Study the drawing (mm; zero at the part's minimum x, y, z) and answer. A direction names the side the tool comes from. Coordinates: 2 decimals unless noted, no trailing zeros. Order: outer loops, then holes, each group sorted by start corner. A loop starts at its lowest first (then second) coordinate and runs counter-clockwise, first axis right, second up.
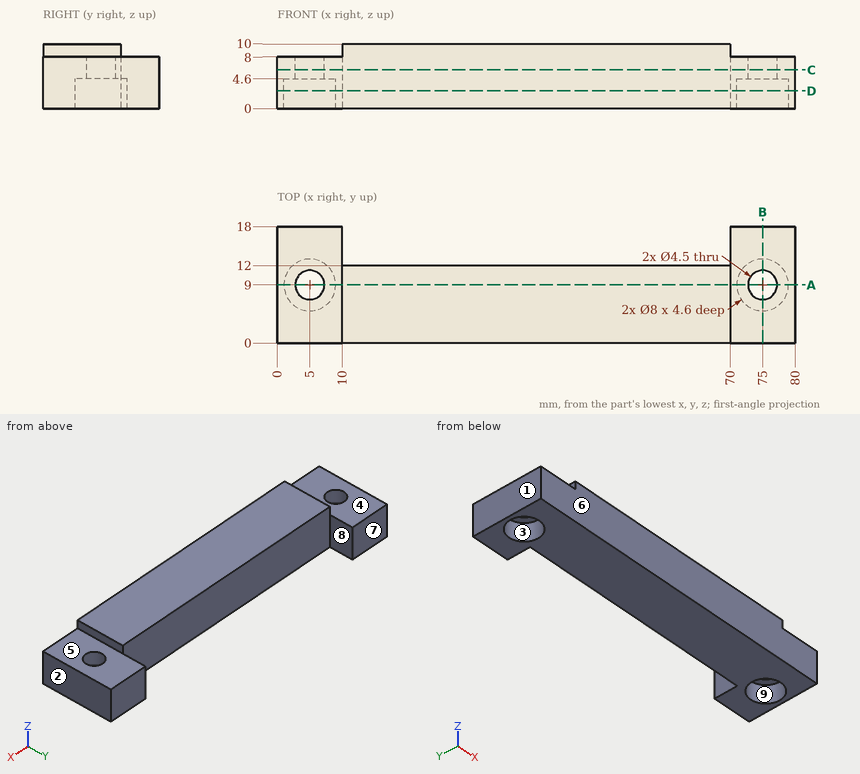
1) A cutting plane is placed at B-B, the plane x = 75. Determine the outline of the cut face in (y, z), and give its area (3 significant figures).
A:
outline: (0, 0) - (5, 0) - (5, 4.6) - (6.75, 4.6) - (6.75, 8) - (0, 8) - close; (11.25, 4.6) - (13, 4.6) - (13, 0) - (18, 0) - (18, 8) - (11.25, 8) - close
area: 91.9 mm2
2) A cutting plane is placed at C-C, the plane z = 6. Determine the outline of the cut face in (x, y).
A:
outline: (0, 0) - (80, 0) - (80, 18) - (70, 18) - (70, 12) - (10, 12) - (10, 18) - (0, 18) - close; hole circle Ø4.5 at (5, 9); hole circle Ø4.5 at (75, 9)
3) Straight lines are drawn through the part: line 1 (X direction, y = 9, z = 7.3); line 2 (X direction, y = 9.25, z = 2.5); line 3 (Y direction, x = 75, z = 7). For each, find the intervals that lie inside material, in ascending order.
A:
line 1: x = 0 to 2.75, 7.25 to 72.75, 77.25 to 80
line 2: x = 0 to 1.01, 8.99 to 71.01, 78.99 to 80
line 3: y = 0 to 6.75, 11.25 to 18
4) Which of the six approach directions +Z, -Z, +X, -X, +Y, -Y give full straight-line access (tool end or side, diameter ignored) to the marked faces 5, 6, 7, 8 and 9?
A:
face 5: +Z, +X, +Y, -Y
face 6: +Z, -Z, +X, -X, -Y
face 7: +Z, -Z, +X, -X, +Y
face 8: +Z, -Z, +Y
face 9: -Z
5) Determine the mould class of the marked faces 1, 2, 3 and 4 for opening direction X: pulls with the +X half, pulls with the -X half, needs draft (parallel to the pull), parting line crosses it, or undercut.
A:
face 1: pulls with the -X half
face 2: pulls with the +X half
face 3: undercut
face 4: needs draft
6) A cutting plane is placed at A-A, the plane y = 9. Determine the outline of the cut face in (x, z), and give its area (3 significant figures).
A:
outline: (0, 0) - (1, 0) - (1, 4.6) - (2.75, 4.6) - (2.75, 8) - (0, 8) - close; (7.25, 4.6) - (9, 4.6) - (9, 0) - (71, 0) - (71, 4.6) - (72.75, 4.6) - (72.75, 8) - (70, 8) - (70, 10) - (10, 10) - (10, 8) - (7.25, 8) - close; (77.25, 4.6) - (79, 4.6) - (79, 0) - (80, 0) - (80, 8) - (77.25, 8) - close
area: 656 mm2
7) Flat-ended cylindrical pins translate along their axes: pin 1 Ø0.6 at (y, z) = (8.5, 9) entering from -X; pin 2 Ø3 at (x, z) = (38, 7) entering from +Y; pin 3 Ø5 at (x, y) = (5, 9) entering from -Z; pin 4 Ø4 at (y, z) = (10.5, 7.5) entering from -X. Find the tip coordinate at first contact, or state that the pin passes through.
A:
pin 1: stops at x = 10
pin 2: stops at y = 12
pin 3: stops at z = 4.6
pin 4: stops at x = 0
8) A cutting plane is placed at D-D, the plane z = 2.75. Determine the outline of the cut face in (x, y).
A:
outline: (0, 0) - (80, 0) - (80, 18) - (70, 18) - (70, 12) - (10, 12) - (10, 18) - (0, 18) - close; hole circle Ø8 at (5, 9); hole circle Ø8 at (75, 9)
